Verification items for the finished model (mm, model axes). Round coordinates to 2 decimals unless told otherwise and drop trailing zeros. Write each loop counter-clockwise with the first axis right and the second up, starting at its lowest first coordinate (ties: lowest second). Pieces come first, ordered by that corner, then holes.
from build123d import *

# Parameters (mm, degrees)
F1_DEPTH = 6.35
F3_DEPTH = 6.351


with BuildPart() as f1:
    # F0 (on Front) → F1 (new body)
    with BuildSketch(Plane.XZ):
        with BuildLine():
            ThreePointArc((-31.75, -52.07), (-31.006051, -53.866051), (-29.21, -54.61))
            Line((-29.21, -54.61), (29.21, -54.61))
            ThreePointArc((29.21, -54.61), (31.006051, -53.866051), (31.75, -52.07))
            Line((31.75, -52.07), (31.75, 52.07))
            ThreePointArc((31.75, 52.07), (31.006051, 53.866051), (29.21, 54.61))
            Line((29.21, 54.61), (-29.21, 54.61))
            ThreePointArc((-29.21, 54.61), (-31.006051, 53.866051), (-31.75, 52.07))
            Line((-31.75, 52.07), (-31.75, -52.07))
        make_face()
    extrude(amount=F1_DEPTH)

    # F2 (on face) → F3 (cut, through all)
    with BuildSketch(Plane.XZ.offset(6.35)):
        with BuildLine():
            Line((-29.4513, 39.751), (-2.5527, 39.751))
            ThreePointArc((-2.5527, 39.751), (-2.103687, 39.936987), (-1.9177, 40.386))
            Line((-1.9177, 40.386), (-1.9177, 52.578))
            ThreePointArc((-1.9177, 52.578), (-2.103687, 53.027013), (-2.5527, 53.213))
            Line((-2.5527, 53.213), (-29.4513, 53.213))
            ThreePointArc((-29.4513, 53.213), (-29.900313, 53.027013), (-30.0863, 52.578))
            Line((-30.0863, 52.578), (-30.0863, 40.386))
            ThreePointArc((-30.0863, 40.386), (-29.900313, 39.936987), (-29.4513, 39.751))
        make_face()
        with BuildLine():
            Line((-30.0863, 37.084), (-30.0863, 24.892))
            ThreePointArc((-30.0863, 24.892), (-29.900313, 24.442987), (-29.4513, 24.257))
            Line((-29.4513, 24.257), (-2.5527, 24.257))
            ThreePointArc((-2.5527, 24.257), (-2.103687, 24.442987), (-1.9177, 24.892))
            Line((-1.9177, 24.892), (-1.9177, 37.084))
            ThreePointArc((-1.9177, 37.084), (-2.103687, 37.533013), (-2.5527, 37.719))
            Line((-2.5527, 37.719), (-29.4513, 37.719))
            ThreePointArc((-29.4513, 37.719), (-29.900313, 37.533013), (-30.0863, 37.084))
        make_face()
        with BuildLine():
            Line((-30.0863, 21.59), (-30.0863, 9.398))
            ThreePointArc((-30.0863, 9.398), (-29.900313, 8.948987), (-29.4513, 8.763))
            Line((-29.4513, 8.763), (-2.5527, 8.763))
            ThreePointArc((-2.5527, 8.763), (-2.103687, 8.948987), (-1.9177, 9.398))
            Line((-1.9177, 9.398), (-1.9177, 21.59))
            ThreePointArc((-1.9177, 21.59), (-2.103687, 22.039013), (-2.5527, 22.225))
            Line((-2.5527, 22.225), (-29.4513, 22.225))
            ThreePointArc((-29.4513, 22.225), (-29.900313, 22.039013), (-30.0863, 21.59))
        make_face()
        with BuildLine():
            Line((-30.0863, 6.096), (-30.0863, -6.096))
            ThreePointArc((-30.0863, -6.096), (-29.900313, -6.545013), (-29.4513, -6.731))
            Line((-29.4513, -6.731), (-2.5527, -6.731))
            ThreePointArc((-2.5527, -6.731), (-2.103687, -6.545013), (-1.9177, -6.096))
            Line((-1.9177, -6.096), (-1.9177, 6.096))
            ThreePointArc((-1.9177, 6.096), (-2.103687, 6.545013), (-2.5527, 6.731))
            Line((-2.5527, 6.731), (-29.4513, 6.731))
            ThreePointArc((-29.4513, 6.731), (-29.900313, 6.545013), (-30.0863, 6.096))
        make_face()
        with BuildLine():
            Line((-30.0863, -9.398), (-30.0863, -21.59))
            ThreePointArc((-30.0863, -21.59), (-29.900313, -22.039013), (-29.4513, -22.225))
            Line((-29.4513, -22.225), (-2.5527, -22.225))
            ThreePointArc((-2.5527, -22.225), (-2.103687, -22.039013), (-1.9177, -21.59))
            Line((-1.9177, -21.59), (-1.9177, -9.398))
            ThreePointArc((-1.9177, -9.398), (-2.103687, -8.948987), (-2.5527, -8.763))
            Line((-2.5527, -8.763), (-29.4513, -8.763))
            ThreePointArc((-29.4513, -8.763), (-29.900313, -8.948987), (-30.0863, -9.398))
        make_face()
        with BuildLine():
            Line((-30.0863, -24.892), (-30.0863, -37.084))
            ThreePointArc((-30.0863, -37.084), (-29.900313, -37.533013), (-29.4513, -37.719))
            Line((-29.4513, -37.719), (-2.5527, -37.719))
            ThreePointArc((-2.5527, -37.719), (-2.103687, -37.533013), (-1.9177, -37.084))
            Line((-1.9177, -37.084), (-1.9177, -24.892))
            ThreePointArc((-1.9177, -24.892), (-2.103687, -24.442987), (-2.5527, -24.257))
            Line((-2.5527, -24.257), (-29.4513, -24.257))
            ThreePointArc((-29.4513, -24.257), (-29.900313, -24.442987), (-30.0863, -24.892))
        make_face()
        with BuildLine():
            Line((-30.0863, -40.386), (-30.0863, -52.578))
            ThreePointArc((-30.0863, -52.578), (-29.900313, -53.027013), (-29.4513, -53.213))
            Line((-29.4513, -53.213), (-2.5527, -53.213))
            ThreePointArc((-2.5527, -53.213), (-2.103687, -53.027013), (-1.9177, -52.578))
            Line((-1.9177, -52.578), (-1.9177, -40.386))
            ThreePointArc((-1.9177, -40.386), (-2.103687, -39.936987), (-2.5527, -39.751))
            Line((-2.5527, -39.751), (-29.4513, -39.751))
            ThreePointArc((-29.4513, -39.751), (-29.900313, -39.936987), (-30.0863, -40.386))
        make_face()
        with BuildLine():
            Line((1.9177, 52.578), (1.9177, 40.386))
            ThreePointArc((1.9177, 40.386), (2.103687, 39.936987), (2.5527, 39.751))
            Line((2.5527, 39.751), (29.4513, 39.751))
            ThreePointArc((29.4513, 39.751), (29.900313, 39.936987), (30.0863, 40.386))
            Line((30.0863, 40.386), (30.0863, 52.578))
            ThreePointArc((30.0863, 52.578), (29.900313, 53.027013), (29.4513, 53.213))
            Line((29.4513, 53.213), (2.5527, 53.213))
            ThreePointArc((2.5527, 53.213), (2.103687, 53.027013), (1.9177, 52.578))
        make_face()
        with BuildLine():
            Line((1.9177, 37.084), (1.9177, 24.892))
            ThreePointArc((1.9177, 24.892), (2.103687, 24.442987), (2.5527, 24.257))
            Line((2.5527, 24.257), (29.4513, 24.257))
            ThreePointArc((29.4513, 24.257), (29.900313, 24.442987), (30.0863, 24.892))
            Line((30.0863, 24.892), (30.0863, 37.084))
            ThreePointArc((30.0863, 37.084), (29.900313, 37.533013), (29.4513, 37.719))
            Line((29.4513, 37.719), (2.5527, 37.719))
            ThreePointArc((2.5527, 37.719), (2.103687, 37.533013), (1.9177, 37.084))
        make_face()
        with BuildLine():
            Line((1.9177, 21.59), (1.9177, 9.398))
            ThreePointArc((1.9177, 9.398), (2.103687, 8.948987), (2.5527, 8.763))
            Line((2.5527, 8.763), (29.4513, 8.763))
            ThreePointArc((29.4513, 8.763), (29.900313, 8.948987), (30.0863, 9.398))
            Line((30.0863, 9.398), (30.0863, 21.59))
            ThreePointArc((30.0863, 21.59), (29.900313, 22.039013), (29.4513, 22.225))
            Line((29.4513, 22.225), (2.5527, 22.225))
            ThreePointArc((2.5527, 22.225), (2.103687, 22.039013), (1.9177, 21.59))
        make_face()
        with BuildLine():
            Line((1.9177, 6.096), (1.9177, -6.096))
            ThreePointArc((1.9177, -6.096), (2.103687, -6.545013), (2.5527, -6.731))
            Line((2.5527, -6.731), (29.4513, -6.731))
            ThreePointArc((29.4513, -6.731), (29.900313, -6.545013), (30.0863, -6.096))
            Line((30.0863, -6.096), (30.0863, 6.096))
            ThreePointArc((30.0863, 6.096), (29.900313, 6.545013), (29.4513, 6.731))
            Line((29.4513, 6.731), (2.5527, 6.731))
            ThreePointArc((2.5527, 6.731), (2.103687, 6.545013), (1.9177, 6.096))
        make_face()
        with BuildLine():
            Line((1.9177, -9.398), (1.9177, -21.59))
            ThreePointArc((1.9177, -21.59), (2.103687, -22.039013), (2.5527, -22.225))
            Line((2.5527, -22.225), (29.4513, -22.225))
            ThreePointArc((29.4513, -22.225), (29.900313, -22.039013), (30.0863, -21.59))
            Line((30.0863, -21.59), (30.0863, -9.398))
            ThreePointArc((30.0863, -9.398), (29.900313, -8.948987), (29.4513, -8.763))
            Line((29.4513, -8.763), (2.5527, -8.763))
            ThreePointArc((2.5527, -8.763), (2.103687, -8.948987), (1.9177, -9.398))
        make_face()
        with BuildLine():
            Line((1.9177, -24.892), (1.9177, -37.084))
            ThreePointArc((1.9177, -37.084), (2.103687, -37.533013), (2.5527, -37.719))
            Line((2.5527, -37.719), (29.4513, -37.719))
            ThreePointArc((29.4513, -37.719), (29.900313, -37.533013), (30.0863, -37.084))
            Line((30.0863, -37.084), (30.0863, -24.892))
            ThreePointArc((30.0863, -24.892), (29.900313, -24.442987), (29.4513, -24.257))
            Line((29.4513, -24.257), (2.5527, -24.257))
            ThreePointArc((2.5527, -24.257), (2.103687, -24.442987), (1.9177, -24.892))
        make_face()
        with BuildLine():
            Line((1.9177, -40.386), (1.9177, -52.578))
            ThreePointArc((1.9177, -52.578), (2.103687, -53.027013), (2.5527, -53.213))
            Line((2.5527, -53.213), (29.4513, -53.213))
            ThreePointArc((29.4513, -53.213), (29.900313, -53.027013), (30.0863, -52.578))
            Line((30.0863, -52.578), (30.0863, -40.386))
            ThreePointArc((30.0863, -40.386), (29.900313, -39.936987), (29.4513, -39.751))
            Line((29.4513, -39.751), (2.5527, -39.751))
            ThreePointArc((2.5527, -39.751), (2.103687, -39.936987), (1.9177, -40.386))
        make_face()
    extrude(amount=-F3_DEPTH, mode=Mode.SUBTRACT)


solid = f1.part
Q1. Sectioned sample at A-A (z = 29). Enter the section's corners in (x, y), plus the area to 3 significant figures.
Recorded:
outline: (-31.75, -6.35) - (-30.09, -6.35) - (-30.09, 0) - (-31.75, 0) - close; (-1.92, -6.35) - (1.92, -6.35) - (1.92, 0) - (-1.92, 0) - close; (30.09, -6.35) - (31.75, -6.35) - (31.75, 0) - (30.09, 0) - close
area: 45.5 mm2
Q2. Sectioned sample at B-B (x = 25.5). Give the number of separate pieces and of enclosed holes in the cut face, plus the area to 3 significant figures.
Recorded:
separate pieces: 8
enclosed holes: 0
area: 95.2 mm2
Q3. Release check for a two-part mould opening along Z. For faces 1 (the cylindrical face through (30.986, -3.131, -53.886)), 2 (the flat face through (16, -3, 6.731)) record: released by +Z, released by -Z, zero draft, split by the parting line, or undercut.
Recorded:
face 1: released by -Z
face 2: undercut
Q4. Material ranges on line 1 along X through (y, z) = (-1, 12.5); line 2 along X through (y, z) = (-2.75, 22), recorded low to high.
Recorded:
line 1: x = -31.75 to -30.09, -1.92 to 1.92, 30.09 to 31.75
line 2: x = -31.75 to -29.94, -2.07 to 2.07, 29.94 to 31.75
